```python
from build123d import *

# Parameters (mm, degrees)
BASPROSKE_W         = 3
BASPROSKE_H         = 24
TOOTHCUT_DEPTH      = 35.073450075
TEETHCUTS_COUNT     = 10
TEETHCUTS_ANGLE     = 324
BORSKE_R            = 5
BORE_DEPTH          = 50.0000508
CUT_EXTRUDE1_DEPTH  = 10
BOSS_EXTRUDE1_DEPTH = 3
FILLET1_R           = 10
FILLET2_R           = 0.5
SKETCH4_R           = 0.723099704
SKETCH4_R_2         = 0.723
CUT_EXTRUDE2_DEPTH  = 60.377084251


with BuildPart() as part:
    # BasProSke → Base-Revolve (revolve)
    with BuildSketch(Plane(origin=(0, 0, 0), x_dir=(1, 0, 0), z_dir=(0, 1, 0)), mode=Mode.PRIVATE) as base_revolve_sk:
        with Locations((1.5, 12)):
            Rectangle(BASPROSKE_W, BASPROSKE_H)
    revolve(base_revolve_sk.sketch.rotate(Axis((-10, 0, 0), (1, 0, 0)), 180), axis=Axis((-10, 0, 0), (1, 0, 0)))

    # TooCutSke → ToothCut (cut, through all)
    with BuildSketch(Plane(origin=(0, 0, 0), x_dir=(0, 0, -1), z_dir=(1, 0, 0))):
        with BuildLine():
            ThreePointArc((2.33803632, 14.815653451), (0, 14.999), (-2.33803632, 14.815653451))
            ThreePointArc((-2.33803632, 14.815653451), (-3.315013319, 19.654913653), (-6.946609122, 22.999227528))
            ThreePointArc((-6.946609122, 22.999227528), (0, 24.0254), (6.946609122, 22.999227528))
            ThreePointArc((6.946609122, 22.999227528), (3.315013319, 19.654913653), (2.33803632, 14.815653451))
        make_face()
    toothcut = extrude(amount=TOOTHCUT_DEPTH, mode=Mode.SUBTRACT)

    # TeethCuts: ToothCut ×10 about axis
    teethcuts_axis = Axis((-10, 0, 0), (1, 0, 0))
    for i in range(1, TEETHCUTS_COUNT):
        add(toothcut.rotate(teethcuts_axis, i * TEETHCUTS_ANGLE / (TEETHCUTS_COUNT - 1)), mode=Mode.SUBTRACT)

    # BorSke → Bore (cut, symmetric)
    with BuildSketch(Plane(origin=(0, 0, 0), x_dir=(0, 0, -1), z_dir=(1, 0, 0))):
        with Locations(Location((0, 0, 0), (0, 0, 180))):
            Circle(BORSKE_R)
    extrude(amount=BORE_DEPTH, both=True, mode=Mode.SUBTRACT)

    # Sketch2 → Cut-Extrude1 (cut)
    with BuildSketch(Plane(origin=(3, 0, 0), x_dir=(0, 0, -1), z_dir=(1, 0, 0))):
        Polygon((6.816911485, -13.360378693), (2.33803632, -14.815653451), (-0.141133304, -15.621184492), (3.422057866, -26.587559293), (12.21539263, -23.730431632), (8.652201461, -12.764056831), align=None)
    extrude(amount=-CUT_EXTRUDE1_DEPTH, mode=Mode.SUBTRACT)

    # Sketch3 → Boss-Extrude1 (add)
    with BuildSketch(Plane(origin=(3, 0, 0), x_dir=(0, 0, -1), z_dir=(1, 0, 0))):
        Polygon((16.145202329, -42.069905854), (12.47904632, -54.349791311), (8.765627157, -53.241151167), (11.666327165, -43.525180612), align=None)
        Polygon((11.666327165, -43.525180612), (16.145202329, -42.069905854), (6.816911485, -13.360378693), (2.33803632, -14.815653451), align=None)
    extrude(amount=-BOSS_EXTRUDE1_DEPTH)

    # Fillet1
    fillet1_edges = [part.edges().sort_by_distance(p)[0] for p in [
        (1.5, -42.069905854, -16.145202329),
        (1.5, -43.525180612, -11.666327165),
    ]]
    fillet(fillet1_edges, radius=FILLET1_R)

    # Fillet2
    fillet2_edges = [part.edges().sort_by_distance(p)[0] for p in [
        (1.5, -54.349791311, -12.47904632),
        (1.5, -53.241151167, -8.765627157),
    ]]
    fillet(fillet2_edges, radius=FILLET2_R)

    # Sketch4 → Cut-Extrude2 (cut, through all)
    with BuildSketch(Plane.ZY):
        with Locations((7.499935211, 0.031174107)):
            Circle(SKETCH4_R)
        with Locations((10.499909296, 0.04364375)):
            Circle(SKETCH4_R_2)
        with Locations((13.499883381, 0.056113393)):
            Circle(SKETCH4_R_2)
        with Locations((-7.499935211, -0.031174107)):
            Circle(SKETCH4_R_2)
        with Locations((-10.499909296, -0.04364375)):
            Circle(SKETCH4_R_2)
        with Locations((-13.462606147, 0)):
            Circle(SKETCH4_R_2)
    extrude(amount=-CUT_EXTRUDE2_DEPTH, mode=Mode.SUBTRACT)


solid = part.part
```
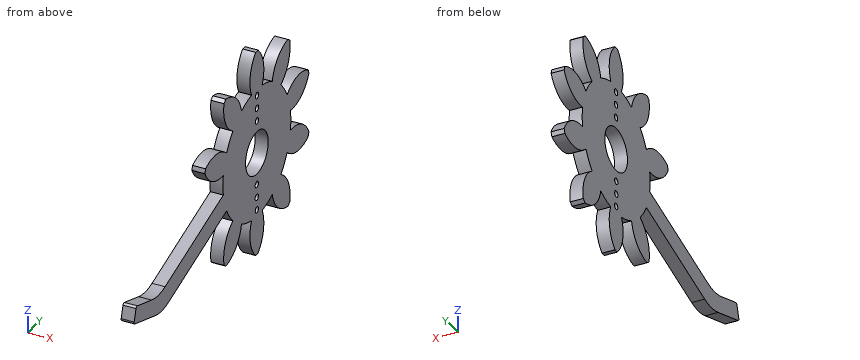
Build history of the part. All positions in model axes, mm. Coordinates: 2 decimals unless noted, no trailing zeros. Write each loop counter-clockwise with the first axis right and the second up, starting at its lowest first coordinate (ties: lowest second). Pieces come first, ordered by that corner, then holes.
1. Band-saw the part on C-C, the plane z = 18. Give the cut face in (x, y).
Answer block:
outline: (0, -14.67) - (3, -14.67) - (3, -9.61) - (0, -9.61) - close; (0, -3.08) - (3, -3.08) - (3, 3.08) - (0, 3.08) - close; (0, 9.61) - (3, 9.61) - (3, 14.67) - (0, 14.67) - close
2. Band-saw the part on B-B, the plane y = 18.5. Give the cut face in (x, z), and give its area (3 significant figures).
Answer block:
outline: (0, -8.92) - (3, -8.92) - (3, -2.78) - (0, -2.78) - close; (0, 2.78) - (3, 2.78) - (3, 8.92) - (0, 8.92) - close
area: 36.8 mm2
3. Drill centre lines: probe 1 along Z at (x, y) = (2.25, -13); probe 2 along Y at (x, z) = (2.6, -18.5); probe 3 along Y at (x, z) = (0.9, -19). Where is each one in solid material? Low to high.
Answer block:
probe 1: z = -19.61 to -12.66, -7.48 to 7.48, 12.66 to 19.61
probe 2: y = -14.62 to -10.3, -3.07 to 3.07, 10.3 to 14.62
probe 3: y = -14.55 to -11.2, -3.03 to 3.03, 11.2 to 14.55
4. Drop flat-ended pins along their axis: pin 1 (2.5 mm diameter, centred on y = 0, z = -13.46, fed in from -X); pin 2 (0.9 mm diameter, centred on y = 0.03, z = 7.5, fed in from +X); pin 3 (1.5 mm diameter, centred on x = 2.5, y = 1.5, fed in from -Z). Give the stop position or say it passes through.
Answer block:
pin 1: stops at x = 0
pin 2: passes through
pin 3: stops at z = -23.78
5. Band-saw the part on D-D, the plane x = 1. Give the number of separate pieces and of enclosed holes in the cut face, and give its area (3 significant figures).
Answer block:
separate pieces: 1
enclosed holes: 7
area: 1,210 mm2
6. Band-saw the part on A-A, the plane z = 0. Give the cut face in (x, y), and give its area (3 significant figures).
Answer block:
outline: (0, -15) - (3, -15) - (3, -5) - (0, -5) - close; (0, 5) - (3, 5) - (3, 15) - (0, 15) - close
area: 60.0 mm2
